from build123d import *

# Parameters (mm, degrees)
SKETCH1_R                = 8
SKETCH1_R_2              = 4
BOSS_EXTRUDE1_DEPTH      = 9
BOSS_EXTRUDE1_2_DEPTH    = 9
SKETCH2_R                = 4
BOSS_EXTRUDE3_DEPTH      = 9
FILLET1_R                = 1
CUT_EXTRUDE1_DEPTH       = 214.789616212
SKETCH4_W                = 9
SKETCH4_H                = 27
BOSS_EXTRUDE4_DEPTH      = 75
BOSS_EXTRUDE5_START      = 9
SKETCH5_R                = 25
SKETCH5_R_2              = 4
BOSS_EXTRUDE5_DEPTH      = 9
BOSS_EXTRUDE6_DEPTH      = 4.5
BOSS_EXTRUDE6_DEPTH_BACK = 4.5
BOSS_EXTRUDE7_DEPTH      = 4.5
BOSS_EXTRUDE7_DEPTH_BACK = 4.5
BOSS_EXTRUDE7_START      = -25
SKETCH9_W                = 9
SKETCH9_H                = 7
SKETCH9_H_2              = 9
CUT_EXTRUDE2_DEPTH       = 217.612557346


with BuildPart() as part:
    # Sketch1 → Boss-Extrude1 (new body)
    with BuildSketch(Plane.XY):
        with Locations((-125, 0)):
            Circle(SKETCH1_R)
        with Locations((-125, 0)):
            Circle(SKETCH1_R_2, mode=Mode.SUBTRACT)
    extrude(amount=BOSS_EXTRUDE1_DEPTH)



with BuildPart() as body_2:
    # Sketch1 → Boss-Extrude1 2 (new body)
    with BuildSketch(Plane.XY):
        with Locations((125, 0)):
            Circle(SKETCH1_R)
        with Locations((125, 0)):
            Circle(SKETCH1_R_2, mode=Mode.SUBTRACT)
    extrude(amount=BOSS_EXTRUDE1_2_DEPTH)


with BuildPart() as part_1:
    add(part.part)

    add(body_2.part)  # Boss-Extrude3 merges body 2
    # Sketch2 → Boss-Extrude3 (add)
    with BuildSketch(Plane.XY):
        with BuildLine():
            Line((-175, -75), (125, -75))
            ThreePointArc((125, -75), (130.131670325, -43.377223009), (145.000000492, -14.999999344))
            ThreePointArc((145.000000492, -14.999999344), (143.981414944, 16.269784471), (113.235294528, 22.058823748))
            ThreePointArc((113.235294528, 22.058823748), (25.000000075, 0), (-63.235294395, 22.058823677))
            ThreePointArc((-63.235294395, 22.058823677), (-75.420498385, 24.996463372), (-87.499999896, 21.650635154))
            ThreePointArc((-87.499999896, 21.650635154), (-99.999999954, 18.301270189), (-112.500000024, 21.650635108))
            ThreePointArc((-112.500000024, 21.650635108), (-124.99999995, 25), (-137.49999989, 21.650635158))
            ThreePointArc((-137.49999989, 21.650635158), (-149.999999954, 18.301270189), (-162.50000003, 21.650635112))
            ThreePointArc((-162.50000003, 21.650635112), (-193.705072901, 16.586749162), (-195.000000551, -14.999999265))
            ThreePointArc((-195.000000551, -14.999999265), (-180.13167034, -43.377222962), (-175, -75))
        make_face()
        with Locations((125, 0)):
            Circle(SKETCH2_R, mode=Mode.SUBTRACT)
        with Locations((-175, 0)):
            Circle(SKETCH2_R, mode=Mode.SUBTRACT)
        with Locations((-125, 0)):
            Circle(SKETCH2_R, mode=Mode.SUBTRACT)
        with Locations((-75, 0)):
            Circle(SKETCH2_R, mode=Mode.SUBTRACT)
    extrude(amount=BOSS_EXTRUDE3_DEPTH)

    # Fillet1
    fillet1_edges = [part_1.edges().sort_by_distance(p)[0] for p in [
        (-175, -75, 4.5),
        (125, -75, 4.5),
    ]]
    fillet(fillet1_edges, radius=FILLET1_R)

    # Sketch3 → Cut-Extrude1 (cut, through all)
    with BuildSketch(Plane.XY):
        Polygon((25, 0), (25, -75), (150, -75), (150, 25), (25, 25), align=None)
    extrude(amount=CUT_EXTRUDE1_DEPTH, mode=Mode.SUBTRACT)

    # Sketch4 → Boss-Extrude4 (add)
    with BuildSketch(Plane.XZ.offset(75)):
        with Locations((25, -4.5)):
            Rectangle(SKETCH4_W, SKETCH4_H)
    extrude(amount=-BOSS_EXTRUDE4_DEPTH)

    # Sketch5 → Boss-Extrude5 (add)
    # profile 1 of 4: a face of its own
    with BuildSketch(Plane(origin=(0, 0, -18), x_dir=(-1, 0, 0), z_dir=(0, 0, -1)).offset(BOSS_EXTRUDE5_START)):
        with BuildLine():
            ThreePointArc((-145.000000304, -14.999999594), (-130.131670275, -43.377223158), (-125, -75))
            Line((-125, -75), (-29.5, -75))
            Line((-29.5, -75), (-29.5, 0))
            Line((-29.5, 0), (-100, 0))
            ThreePointArc((-100, 0), (-117.09430609, -23.717082532), (-145.000000304, -14.999999594))
        make_face()
    # profile 2 of 4: a face of its own
    with BuildSketch(Plane(origin=(0, 0, -18), x_dir=(-1, 0, 0), z_dir=(0, 0, -1)).offset(BOSS_EXTRUDE5_START)):
        with Locations((-125, 0)):
            Circle(SKETCH5_R)
        with Locations((-125, 0)):
            Circle(SKETCH5_R_2, mode=Mode.SUBTRACT)
    # profile 3 of 4: a face of its own
    with BuildSketch(Plane(origin=(0, 0, -18), x_dir=(-1, 0, 0), z_dir=(0, 0, -1)).offset(BOSS_EXTRUDE5_START)):
        Polygon((-29.5, 0), (-29.5, -75), (-20.5, -75), (-20.5, 0), (-25, 0), align=None)
    # profile 4 of 4: a face of its own
    with BuildSketch(Plane(origin=(0, 0, -18), x_dir=(-1, 0, 0), z_dir=(0, 0, -1)).offset(BOSS_EXTRUDE5_START)):
        with BuildLine():
            Line((-100, 0), (-29.5, 0))
            Line((-29.5, 0), (-25, 0))
            ThreePointArc((-25, 0), (-70.475429529, 5.598281181), (-113.235293817, 22.058823369))
            ThreePointArc((-113.235293817, 22.058823369), (-103.56267677, 12.86239374), (-100, 0))
        make_face()
    extrude(amount=-BOSS_EXTRUDE5_DEPTH)

    # Sketch7 → Boss-Extrude6 (add, two sides: drawn at the far end of the back side and taken through both)
    with BuildSketch(Plane(origin=(0, -25, 0), x_dir=(1, 0, 0), z_dir=(0, 1, 0)).offset(-BOSS_EXTRUDE6_DEPTH_BACK)):
        with BuildLine():
            Line((56.5, 18), (29.5, 18))
            Line((29.5, 18), (29.5, -9))
            ThreePointArc((29.5, -9), (48.591883092, -1.091883092), (56.5, 18))
        make_face()
        with BuildLine():
            Line((-6.5, 0), (20.5, 0))
            Line((20.5, 0), (20.5, 27))
            ThreePointArc((20.5, 27), (1.408116908, 19.091883092), (-6.5, 0))
        make_face()
    extrude(amount=BOSS_EXTRUDE6_DEPTH + BOSS_EXTRUDE6_DEPTH_BACK)

    # Sketch7<3> → Boss-Extrude7 (add, two sides: drawn at the far end of the back side and taken through both)
    with BuildSketch(Plane(origin=(0, -25, 0), x_dir=(1, 0, 0), z_dir=(0, 1, 0)).offset(BOSS_EXTRUDE7_START - BOSS_EXTRUDE7_DEPTH_BACK)):
        with BuildLine():
            Line((56.5, 18), (29.5, 18))
            Line((29.5, 18), (29.5, -9))
            ThreePointArc((29.5, -9), (48.591883092, -1.091883092), (56.5, 18))
        make_face()
        with BuildLine():
            Line((-6.5, 0), (20.5, 0))
            Line((20.5, 0), (20.5, 27))
            ThreePointArc((20.5, 27), (1.408116908, 19.091883092), (-6.5, 0))
        make_face()
    extrude(amount=BOSS_EXTRUDE7_DEPTH + BOSS_EXTRUDE7_DEPTH_BACK)

    # Sketch9 → Cut-Extrude2 (cut, through all)
    with BuildSketch(Plane.XY.offset(9)):
        with Locations((-160.208548161, -53.5)):
            Rectangle(SKETCH9_W, SKETCH9_H)
        with Locations((-160.208548161, -70.5)):
            Rectangle(SKETCH9_W, SKETCH9_H_2)
        with Locations((-25.351798772, -53.5)):
            Rectangle(SKETCH9_W, SKETCH9_H)
        with Locations((-25.351798772, -70.5)):
            Rectangle(SKETCH9_W, SKETCH9_H_2)
        with Locations((109.504950616, -53.5)):
            Rectangle(SKETCH9_W, SKETCH9_H)
        with Locations((109.504950616, -70.5)):
            Rectangle(SKETCH9_W, SKETCH9_H_2)
    extrude(amount=-CUT_EXTRUDE2_DEPTH, mode=Mode.SUBTRACT)


solid = part_1.part
The listing builds one solid part. Answer for the finished solid, in the listing's coordinates (mm). A direction names the side the tool comes from. Coordinates: 2 decimals unless noted, no trailing zeros. Order: outer loops, then holes, each group sorted by start corner. A loop starts at its lowest first (then second) coordinate and runs counter-clockwise, first axis right, second up.
Q1. Given P1, Ø1.5, axis at y = -58, z = -20, coming from the -X side; P2, Ø1, axis at x = -9.5, y = -21, coming from the -Z side; P3, Ø10, axis at x = 24.5, z = -6.5, coming from the +Y side, each flat-ended and moving along its own axis, determine where each tip first touches the part or whether it passes through.
Q2. A cutting plane is placed at D-D, the plane x = 61. Write down the section's boundary in (y, z), and give its area (3 significant figures).
Q3. Consider line 1 (X direction, y = -70, z = 7.5); line 2 (Y direction, x = -125, z = 6.75); line 3 (X direction, y = -69.5, z = -3.5). Determine where each line is inside the solid, lowest interval first.
Q4. A cutting plane is placed at B-B, the plane z = -24. Write down the section's boundary in (x, y), and give its area (3 significant figures).
Q5. Which of the six approach directions +Z, -Z, +X, -X, +Y, -Y give full straight-line access (tool end or side, diameter ignored) to faces 1 (the face through (20.5, -10, -14)), 2 (the face through (-155.709, -71, 5)), 3 (the face through (-160, -57, 5)), 4 (the face through (29.5, -65, -5))?
Q6. A cutting plane is placed at C-C, the plane z = -7.5. Write down the section's boundary in (x, y).
Q7. For a pull along X with two mould halves and no side action, classify faces 5 (the face through (-180.43, -42.49, 4.44)), 6 (the face through (-29.852, -71, 5)), 7 (the face through (40, -20.5, -8)) as pulls with the +X half, pulls with the -X half, needs draft (parallel to the pull), parting line crosses it, or undercut.
Q8. A cutting plane is placed at A-A, the plane x = -125. Write down the section's boundary in (y, z).
Answers follow:
1. P1: stops at x = 20.5
1. P2: stops at z = 0
1. P3: stops at y = 0
2. outline: (-75, -27) - (3.49, -27) - (3.49, -18) - (-75, -18) - close
2. area: 706 mm2
3. line 1: x = -175.13 to -164.71, -155.71 to -29.85, -20.85 to 29.5
3. line 2: y = -75 to -4, 4 to 25
3. line 3: x = 20.5 to 29.5
4. outline: (8.13, -54.5) - (20.5, -54.5) - (20.5, -75) - (105, -75) - (105, -66) - (114, -66) - (114, -75) - (125, -75) arc R100 cw to (145, -15) arc R25 ccw to (113.24, 22.06) arc R187.5 cw to (25, 0) - (20.5, 0) - (20.5, -20.5) - (8.13, -20.5) - (8.13, -29.5) - (20.5, -29.5) - (20.5, -45.5) - (8.13, -45.5) - close; hole (105, -57) - (114, -57) - (114, -50) - (105, -50) - close; hole circle Ø8 at (125, 0)
4. area: 10,000 mm2
5. face 1: -Z, -X, +Y
5. face 2: +Z, -Z, -Y
5. face 3: +Z, -Z
5. face 4: +Z, +X, -Y
6. outline: (-5.44, -54.5) - (20.5, -54.5) - (20.5, -75) - (29.5, -75) - (29.5, -54.5) - (54.37, -54.5) - (54.37, -45.5) - (29.5, -45.5) - (29.5, -29.5) - (54.37, -29.5) - (54.37, -20.5) - (29.5, -20.5) - (29.5, 0) - (20.5, 0) - (20.5, -20.5) - (-5.44, -20.5) - (-5.44, -29.5) - (20.5, -29.5) - (20.5, -45.5) - (-5.44, -45.5) - close
7. face 5: pulls with the -X half
7. face 6: undercut
7. face 7: needs draft
8. outline: (-75, 0) - (-4, 0) - (-4, 9) - (-75, 9) - close; (4, 0) - (25, 0) - (25, 9) - (4, 9) - close
